Part model, mm, in its own coordinate system. A direction names the side the tool comes from. Round coordinates to 2 decimals unless told otherwise and drop trailing zeros. Write each loop counter-clockwise with the first axis right and the second up, starting at its lowest first coordinate (ties: lowest second). Pieces come first, ordered by that corner, then holes. Notation, with made-up numbers: M 0,78.25 L 28,78.25 A21 ccw 28,95.25 Z; hole C 24,-12 d3. An arc over 180 degrees is marked long. One line per question, with ' | ' between items. Start each with the question number.
1) Saw through at A-A (z = 13.75). List the corners of the cut face in (x, y).
2) Wall check: probe 1 along X at (y, z) = (2, 14); probe 2 along X at (y, z) = (-4.75, 15.75); probe 3 along Z at (x, y) = (-17.75, -6.5). Give the ranges that are in metal, low to high. Write a range as [from, to].
3) Drop flat-ended pins along their axis: pin 1 Ø3 at (y, z) = (1.5, 8.5) entering from +X; pin 2 Ø6 at (y, z) = (-1, 11) entering from -X; pin 3 Ø3 at (x, y) = (-4.5, -8.5) entering from -Z; pin 4 Ø1.5 at (x, y) = (-16.5, -7.5) entering from +Z. Give the stop position or say it passes through.
4) Tool access for faces 1 (the face through (-5, -3, 20)), 2 (the face through (-16, -5, 5)), 3 (the face through (2.682, -3, 14)): list every direction of +Z, -Z, +X, -X, +Y, -Y with a clear straight run to the whole face (end or side of a thin tool).
5) Saw through at B-B (y = -0.75). List the corners of the cut face in (x, z), plus the area to 3 significant figures.
6) Mould opens along Z. For faces 4 (the face through (-13.07, -3.087, 5.713)), 5 (the face through (-5, -3, 0)), 6 (the face through (-8.79, -3.3, 10.71)), 7 (the face through (-5, 4.308, 8)) say: pulls with the +Z half, pulls with the -Z half, needs draft (parallel to the pull), parting line crosses it, or undercut.
7) Saw through at C-C (x = -1.75). List the corners of the cut face in (y, z).
```python
from build123d import *

# Parameters (mm, degrees)
F0_W      = 30
F0_H      = 15
F1_DEPTH  = 20
F2_W      = 7.5
F2_H      = 15
F3_DEPTH  = 15.001
F4_R      = 2.5
F5_R      = 5
F6_DEPTH  = 15.001
F7_R      = 2
F8_DEPTH  = 5.001
F9_R      = 2
F10_DEPTH = 5.001


with BuildPart() as f1:
    # F0 (on Top) → F1 (new body)
    with BuildSketch(Plane.XY):
        with Locations((-4.818223, -3.192319)):
            Rectangle(F0_W, F0_H)
    extrude(amount=F1_DEPTH)

    # F2 (on face) → F3 (cut, through all)
    with BuildSketch(Plane.XZ.offset(10.692319)):
        with Locations((-16.068223, 12.5)):
            Rectangle(F2_W, F2_H)
        with Locations((6.431777, 12.5)):
            Rectangle(F2_W, F2_H)
    extrude(amount=-F3_DEPTH, mode=Mode.SUBTRACT)

    # F4
    f4_edges = [f1.edges().sort_by_distance(p)[0] for p in [
        (2.681777, -3.192319, 5),
        (-12.318223, -3.192319, 5),
    ]]
    fillet(f4_edges, radius=F4_R)

    # F5 (on face) → F6 (cut, through all)
    with BuildSketch(Plane.XZ.offset(10.692319)):
        with Locations((-4.818223, 13.75)):
            Circle(F5_R)
    extrude(amount=-F6_DEPTH, mode=Mode.SUBTRACT)

    # F7 (on face) → F8 (cut, through all)
    with BuildSketch(Plane.XY.offset(5)):
        with Locations((7.681777, -3.192319)):
            Circle(F7_R)
    extrude(amount=-F8_DEPTH, mode=Mode.SUBTRACT)

    # F9 (on face) → F10 (cut, through all)
    with BuildSketch(Plane.XY.offset(5)):
        with Locations((-17.318223, -3.192319)):
            Circle(F9_R)
    extrude(amount=-F10_DEPTH, mode=Mode.SUBTRACT)


solid = f1.part
```
Answer key:
1) outline: M -12.32,-10.69 L -9.82,-10.69 L -9.82,4.31 L -12.32,4.31 Z; M 0.18,-10.69 L 2.68,-10.69 L 2.68,4.31 L 0.18,4.31 Z
2) probe 1: x = [-12.32, -9.81], [0.18, 2.68] | probe 2: x = [-12.32, -9.4], [-0.24, 2.68] | probe 3: z = [0, 5]
3) pin 1: stops at x = 2.73 | pin 2: stops at x = -12.32 | pin 3: stops at z = 0 | pin 4: stops at z = 5
4) face 1: +Z, +X, -X, +Y, -Y | face 2: +Z, -X, +Y, -Y | face 3: +Z, +X, +Y, -Y
5) outline: M -19.82,0 L 10.18,0 L 10.18,5 L 5.18,5 A2.5 cw 2.68,7.5 L 2.68,20 L -12.32,20 L -12.32,7.5 A2.5 cw -14.82,5 L -19.82,5 Z; hole C -4.82,13.75 d10 | area: 299 mm2
6) face 4: pulls with the +Z half | face 5: pulls with the -Z half | face 6: undercut | face 7: needs draft
7) outline: M -10.69,0 L 4.31,0 L 4.31,9.8 L -10.69,9.8 Z; M -10.69,17.7 L 4.31,17.7 L 4.31,20 L -10.69,20 Z
